Could you check a few things on this model? Use its own coordinates, in mm. Coordinates: 2 decimals unless noted, no trailing zeros. Order: outer loops, then holes, each group sorted by start corner. A loop starts at its lowest first (then second) coordinate and runs counter-clockwise, first axis right, second up.
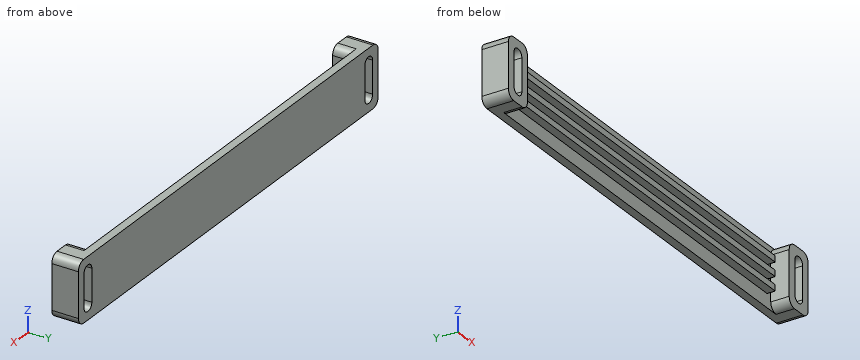
```python
from build123d import *

# Parameters (mm, degrees)
SKETCH_1_W          = 97
SKETCH_1_H          = 1.5
EXTRUDE_1_DEPTH     = 2
EXTRUDE_1_2_DEPTH   = 2
EXTRUDE_1_3_DEPTH   = 2
SKETCH_2_W          = 114.23
SKETCH_2_H          = 15
EXTRUDE_2_DEPTH     = 2
CUT_EXTRUDE_1_DEPTH = 10
FILLET_1_R          = 2
EXTRUDE_3_DEPTH     = 4.54


with BuildPart() as part:
    # Sketch 1 → Extrude 1 (new body)
    with BuildSketch(Plane(origin=(0, 0, 0), x_dir=(1, 0, 0), z_dir=(0, 1, 0))):
        Rectangle(SKETCH_1_W, SKETCH_1_H)
    extrude(amount=EXTRUDE_1_DEPTH)



with BuildPart() as body_2:
    # Sketch 1 → Extrude 1 2 (new body)
    with BuildSketch(Plane(origin=(0, 0, 0), x_dir=(1, 0, 0), z_dir=(0, 1, 0))):
        with Locations((0, -3.4)):
            Rectangle(SKETCH_1_W, SKETCH_1_H)
    extrude(amount=EXTRUDE_1_2_DEPTH)


with BuildPart() as body_3:
    # Sketch 1 → Extrude 1 3 (new body)
    with BuildSketch(Plane(origin=(0, 0, 0), x_dir=(1, 0, 0), z_dir=(0, 1, 0))):
        with Locations((0, -6.8)):
            Rectangle(SKETCH_1_W, SKETCH_1_H)
    extrude(amount=EXTRUDE_1_3_DEPTH)


with BuildPart() as part_1:
    add(part.part)

    add(body_2.part)  # Extrude 2 merges body 2

    add(body_3.part)  # Extrude 2 merges body 3
    # Sketch 2 → Extrude 2 (add)
    with BuildSketch(Plane(origin=(0, 2, 0), x_dir=(1, 0, 0), z_dir=(0, 1, 0))):
        with Locations((0, -3.4)):
            Rectangle(SKETCH_2_W, SKETCH_2_H)
    extrude(amount=EXTRUDE_2_DEPTH)

    # Sketch 3 → Cut-Extrude 1 (cut)
    with BuildSketch(Plane(origin=(0, 4, 0), x_dir=(1, 0, 0), z_dir=(0, 1, 0))):
        with BuildLine():
            Line((-53.5, 2.1), (-53.5, -3.4))
            Line((-53.5, -3.4), (-52, -3.4))
            Line((-52, -3.4), (-52, 0.6))
            ThreePointArc((-52, 0.6), (-52.439339828, 1.660660172), (-53.5, 2.1))
        make_face()
        with BuildLine():
            Line((-55, 0.6), (-55, -3.4))
            Line((-55, -3.4), (-53.5, -3.4))
            Line((-53.5, -3.4), (-53.5, 2.1))
            ThreePointArc((-53.5, 2.1), (-54.560660172, 1.660660172), (-55, 0.6))
        make_face()
        with BuildLine():
            Line((-53.5, -3.4), (-55, -3.4))
            Line((-55, -3.4), (-55, -7.4))
            ThreePointArc((-55, -7.4), (-53.5, -8.9), (-52, -7.4))
            Line((-52, -7.4), (-52, -3.4))
            Line((-52, -3.4), (-53.5, -3.4))
        make_face()
        with BuildLine():
            Line((53.5, -3.4), (52, -3.4))
            Line((52, -3.4), (52, -7.4))
            ThreePointArc((52, -7.4), (53.5, -8.9), (55, -7.4))
            Line((55, -7.4), (55, -3.4))
            Line((55, -3.4), (53.5, -3.4))
        make_face()
        with BuildLine():
            Line((53.5, 2.1), (53.5, -3.4))
            Line((53.5, -3.4), (55, -3.4))
            Line((55, -3.4), (55, 0.6))
            ThreePointArc((55, 0.6), (54.560660172, 1.660660172), (53.5, 2.1))
        make_face()
        with BuildLine():
            Line((52, 0.6), (52, -3.4))
            Line((52, -3.4), (53.5, -3.4))
            Line((53.5, -3.4), (53.5, 2.1))
            ThreePointArc((53.5, 2.1), (52.439339828, 1.660660172), (52, 0.6))
        make_face()
    extrude(amount=-CUT_EXTRUDE_1_DEPTH, mode=Mode.SUBTRACT)

    # Fillet 1
    fillet_1_edges = [part_1.edges().sort_by_distance(p)[0] for p in [
        (57.115, 3, 10.9),
        (57.115, 3, -4.1),
        (-57.115, 3, -4.1),
        (-57.115, 3, 10.9),
    ]]
    fillet(fillet_1_edges, radius=FILLET_1_R)

    # Sketch 4 → Extrude 3 (add)
    # profile 1 of 2: a face of its own
    with BuildSketch(Plane.XZ.offset(-2)):
        with BuildLine():
            Line((55.115, 10.9), (51.885, 10.9))
            ThreePointArc((51.885, 10.9), (50.470786438, 10.314213562), (49.885, 8.9))
            Line((49.885, 8.9), (49.885, -2.1))
            ThreePointArc((49.885, -2.1), (50.470786438, -3.514213562), (51.885, -4.1))
            Line((51.885, -4.1), (55.115, -4.1))
            ThreePointArc((55.115, -4.1), (56.529213562, -3.514213562), (57.115, -2.1))
            Line((57.115, -2.1), (57.115, 8.9))
            ThreePointArc((57.115, 8.9), (56.529213562, 10.314213562), (55.115, 10.9))
        make_face()
        with BuildLine():
            Line((55, 7.4), (55, -0.6))
            ThreePointArc((55, -0.6), (53.5, -2.1), (52, -0.6))
            Line((52, -0.6), (52, 7.4))
            ThreePointArc((52, 7.4), (53.5, 8.9), (55, 7.4))
        make_face(mode=Mode.SUBTRACT)
    # profile 2 of 2: a face of its own
    with BuildSketch(Plane.XZ.offset(-2)):
        with BuildLine():
            Line((-49.885, -2.1), (-49.885, 8.9))
            ThreePointArc((-49.885, 8.9), (-50.470786438, 10.314213562), (-51.885, 10.9))
            Line((-51.885, 10.9), (-55.115, 10.9))
            ThreePointArc((-55.115, 10.9), (-56.529213562, 10.314213562), (-57.115, 8.9))
            Line((-57.115, 8.9), (-57.115, -2.1))
            ThreePointArc((-57.115, -2.1), (-56.529213562, -3.514213562), (-55.115, -4.1))
            Line((-55.115, -4.1), (-51.885, -4.1))
            ThreePointArc((-51.885, -4.1), (-50.470786438, -3.514213562), (-49.885, -2.1))
        make_face()
        with BuildLine():
            ThreePointArc((-55, 7.4), (-53.5, 8.9), (-52, 7.4))
            Line((-52, 7.4), (-52, -0.6))
            ThreePointArc((-52, -0.6), (-53.5, -2.1), (-55, -0.6))
            Line((-55, -0.6), (-55, 7.4))
        make_face(mode=Mode.SUBTRACT)
    extrude(amount=EXTRUDE_3_DEPTH)


solid = part_1.part
```
Item 1: Suppose I cut it at B-B (y = 3). List the corners of the cut face in (x, z) for me (3 decimals).
Item 2: I need wall thicknesses on line 1 (X direction, y = -1, z = 4) (3 decimals); line 2 (X direction, y = 1.75, z = 0.5) (3 decimals); line 3 (Z direction, x = 18, y = 1.5). Which ranges of each line are inside material? Lowest first, please.
Item 3: Suppose I cut it at C-C (x = -28.5). List the corners of the cut face in (y, z) for me.
Item 4: Suppose I cut it at A-A (x = -53.5). List the corners of the cut face in (y, z) for me, and give its area (3 significant figures).
Item 5: For pin 1 Ø1 at (x, z) = (-33.5, 9) entering from -Y; pin 2 Ø1.2 at (x, z) = (-18.5, 3.5) entering from -Y; pin 3 Ø1.6 at (x, y) = (-8.5, 1) entering from +Z, each with a flat end and sliding along its axis, tell me the tip position at first contact or that it passes through.
Geometry results:
1. outline: (-57.115, -2.1) arc R2 ccw to (-55.115, -4.1) - (55.115, -4.1) arc R2 ccw to (57.115, -2.1) - (57.115, 8.9) arc R2 ccw to (55.115, 10.9) - (-55.115, 10.9) arc R2 ccw to (-57.115, 8.9) - close; hole (-55, -0.6) arc R1.5 ccw to (-52, -0.6) - (-52, 7.4) arc R1.5 ccw to (-55, 7.4) - close; hole (52, -0.6) arc R1.5 ccw to (55, -0.6) - (55, 7.4) arc R1.5 ccw to (52, 7.4) - close
2. line 1: x = -57.115 to -55, -52 to -49.885, 49.885 to 52, 55 to 57.115
2. line 2: x = -57.115 to -55, -52 to -49.885, -48.5 to 48.5, 49.885 to 52, 55 to 57.115
2. line 3: z = -0.75 to 0.75, 2.65 to 4.15, 6.05 to 7.55
3. outline: (0, -0.75) - (2, -0.75) - (2, -4.1) - (4, -4.1) - (4, 10.9) - (2, 10.9) - (2, 7.55) - (0, 7.55) - (0, 6.05) - (2, 6.05) - (2, 4.15) - (0, 4.15) - (0, 2.65) - (2, 2.65) - (2, 0.75) - (0, 0.75) - close
4. outline: (-2.54, -4.1) - (4, -4.1) - (4, -2.1) - (-2.54, -2.1) - close; (-2.54, 8.9) - (4, 8.9) - (4, 10.9) - (-2.54, 10.9) - close
4. area: 26.2 mm2
5. pin 1: stops at y = 2
5. pin 2: stops at y = 0
5. pin 3: stops at z = 7.55
